Can you work these out from the model? Positions are in its coordinate system, mm. A direction names the side the tool comes from. Round coordinates to 2 decimals unless told otherwise and drop trailing zeros. Write each loop counter-clockwise with the first axis right and the second up, starting at its lowest first coordinate (ties: lowest second). Pieces come first, ordered by that corner, then holes. Notation, with made-up numbers: M 33,-1.5 L 51,-1.5 A22 cw 51,17.5 Z; hole C 85,86.25 d4. An arc over 180 degrees is marked long. Answer as a JSON object with one key per item and string values. Group by question number.
1) Suppose I cut it at A-A, the plane x = 38.13. Write out the boundary of the cut face in (y, z), and give its area (3 significant figures).
2) Please list where these lines run through material, in increasing order: L1, parallel to Z at x = 41.88, y = 36.4; L2, parallel to X at y = 36, z = 3.75; L3, parallel to Y at x = 35.5, z = 24.25. Write a range as [from, to].
3) Suppose I cut it at B-B, the plane x = 50.5. Write out the boundary of the cut face in (y, z).
4) Suppose I cut it at D-D, the plane y = 28. Write out the boundary of the cut face in (x, z).
5) Suppose I cut it at C-C, the plane z = 14.5. Write out the boundary of the cut face in (x, y).
6) I'm going to push flat-ended pins straight in: pin 1 Ø1 at (y, z) = (9.5, 7) entering from -X; pin 2 Ø1.1 at (x, z) = (22.5, 3.5) entering from +Y; pin 3 Ø5 at (y, z) = (19.5, 18) entering from +X. Where does each tip first touch, or does it pass through?
7) On a 3-axis mill with a long thin cutter (end or side, diameter ignored), from which of +Z, -Z, +X, -X, +Y, -Y can I reach the whole of each face in a straight line? I mean faces 1 (the flat face through (3, 37, 3)), 2 (the flat face through (5, 1, 23)), 3 (the flat face through (17, 36, 6.5)), 4 (the flat face through (65, 1, 26)), 5 (the flat face through (25, 2, 14)). Say none if no direction works.
8) If we mould it in two halves opening along Z, with no side actions, what happens to faces 6 (the flat face through (60, 1, 23)), 7 (the flat face through (0, 1, 2)), 8 (the flat face through (32, 16, 28)), 9 (the cylindrical face through (37.589, 0.507, 22.533))? For each: +Z half, -Z half, draft (parallel to the pull), parting line (faces both ways), or undercut.
from build123d import *

# Parameters (mm, degrees)
SKETCH_1_W           = 65
SKETCH_1_H           = 38
EXTRUDE_1_DEPTH      = 28
SKETCH_2_W           = 30
SKETCH_2_H           = 32
CUT_EXTRUDE_1_DEPTH  = 81.330567034
CUT_EXTRUDE_3_REACH  = 82.331
SKETCH_3_R           = 0.75
SKETCH_4_W           = 15
SKETCH_4_H           = 1.5
CUT_EXTRUDE_4_DEPTH  = 30
SKETCH_5_R           = 11
CUT_EXTRUDE_5_DEPTH  = 81.330567034
CUT_EXTRUDE_6_REACH  = 82.331
SKETCH_6_R           = 0.75
CUT_EXTRUDE_7_REACH  = 82.331
SKETCH_7_W           = 8
SKETCH_7_H           = 24.102688632
SKETCH_8_R           = 1.8
CUT_EXTRUDE_8_DEPTH  = 1
CUT_EXTRUDE_START    = -1
SKETCH_9_R           = 1.8
CUT_EXTRUDE_9_DEPTH  = 1
SKETCH_10_W          = 20
SKETCH_10_H          = 1.7
CUT_EXTRUDE_10_DEPTH = 12


with BuildPart() as part:
    # Sketch 1 → Extrude 1 (new body)
    with BuildSketch(Plane.XY):
        with Locations((32.5, 19)):
            Rectangle(SKETCH_1_W, SKETCH_1_H)
    extrude(amount=EXTRUDE_1_DEPTH)

    # Sketch 2 → Cut-Extrude 1 (cut, through all)
    with BuildSketch(Plane.XY.offset(28)):
        with Locations((15, 19)):
            Rectangle(SKETCH_2_W, SKETCH_2_H)
    cut_extrude_1 = extrude(amount=-CUT_EXTRUDE_1_DEPTH, mode=Mode.SUBTRACT)

    # Sketch 3 → Cut-Extrude 3 (cut, up to next)
    with BuildSketch(Plane(origin=(0, 38, 0), x_dir=(1, 0, 0), z_dir=(0, 1, 0)), mode=Mode.PRIVATE) as cut_extrude_3_sk1:
        with Locations(Location((2.42, -3.75, 0), (0, 0, 270))):
            Circle(SKETCH_3_R)
    cut_extrude_3_tool1 = extrude(cut_extrude_3_sk1.sketch, amount=-CUT_EXTRUDE_3_REACH, mode=Mode.PRIVATE) & part.part
    # Sketch 3 → Cut-Extrude 3 (cut, up to next)
    with BuildSketch(Plane(origin=(0, 38, 0), x_dir=(1, 0, 0), z_dir=(0, 1, 0)), mode=Mode.PRIVATE) as cut_extrude_3_sk2:
        with Locations(Location((23.12, -3.75, 0), (0, 0, 270))):
            Circle(SKETCH_3_R)
    cut_extrude_3_tool2 = extrude(cut_extrude_3_sk2.sketch, amount=-CUT_EXTRUDE_3_REACH, mode=Mode.PRIVATE) & part.part
    # Sketch 3 → Cut-Extrude 3 (cut, up to next)
    with BuildSketch(Plane(origin=(0, 38, 0), x_dir=(1, 0, 0), z_dir=(0, 1, 0)), mode=Mode.PRIVATE) as cut_extrude_3_sk3:
        with Locations(Location((23.12, -24.25, 0), (0, 0, 270))):
            Circle(SKETCH_3_R)
    cut_extrude_3_tool3 = extrude(cut_extrude_3_sk3.sketch, amount=-CUT_EXTRUDE_3_REACH, mode=Mode.PRIVATE) & part.part
    # Sketch 3 → Cut-Extrude 3 (cut, up to next)
    with BuildSketch(Plane(origin=(0, 38, 0), x_dir=(1, 0, 0), z_dir=(0, 1, 0)), mode=Mode.PRIVATE) as cut_extrude_3_sk4:
        with Locations(Location((2.42, -24.25, 0), (0, 0, 270))):
            Circle(SKETCH_3_R)
    cut_extrude_3_tool4 = extrude(cut_extrude_3_sk4.sketch, amount=-CUT_EXTRUDE_3_REACH, mode=Mode.PRIVATE) & part.part
    cut_extrude_3_1 = cut_extrude_3_tool1.solids().sort_by_distance((2.42, 38, 3.75))[0]
    add(cut_extrude_3_1, mode=Mode.SUBTRACT)
    cut_extrude_3_2 = cut_extrude_3_tool2.solids().sort_by_distance((23.12, 38, 3.75))[0]
    add(cut_extrude_3_2, mode=Mode.SUBTRACT)
    cut_extrude_3_3 = cut_extrude_3_tool3.solids().sort_by_distance((23.12, 38, 24.25))[0]
    add(cut_extrude_3_3, mode=Mode.SUBTRACT)
    cut_extrude_3_4 = cut_extrude_3_tool4.solids().sort_by_distance((2.42, 38, 24.25))[0]
    add(cut_extrude_3_4, mode=Mode.SUBTRACT)
    cut_extrude_3 = cut_extrude_3_1 + cut_extrude_3_2 + cut_extrude_3_3 + cut_extrude_3_4  # Cut-Extrude 3 as one shape, for the pattern or mirror that repeats it

    # Sketch 4 → Cut-Extrude 4 (cut)
    with BuildSketch(Plane.ZY):
        with Locations((14, 35.75)):
            Rectangle(SKETCH_4_W, SKETCH_4_H)
    cut_extrude_4 = extrude(amount=-CUT_EXTRUDE_4_DEPTH, mode=Mode.SUBTRACT)

    # Sketch 5 → Cut-Extrude 5 (cut, through all)
    with BuildSketch(Plane(origin=(0, 38, 0), x_dir=(1, 0, 0), z_dir=(0, 1, 0))):
        with Locations((-4.5, -14)):
            Circle(SKETCH_5_R)
    cut_extrude_5 = extrude(amount=-CUT_EXTRUDE_5_DEPTH, mode=Mode.SUBTRACT)

    # Sketch 6 → Cut-Extrude 6 (cut, up to next)
    with BuildSketch(Plane.XZ, mode=Mode.PRIVATE) as cut_extrude_6_sk1:
        with Locations(Location((2.42, 3.75, 0), (0, 0, 90))):
            Circle(SKETCH_6_R)
    cut_extrude_6_tool1 = extrude(cut_extrude_6_sk1.sketch, amount=-CUT_EXTRUDE_6_REACH, mode=Mode.PRIVATE) & part.part
    # Sketch 6 → Cut-Extrude 6 (cut, up to next)
    with BuildSketch(Plane.XZ, mode=Mode.PRIVATE) as cut_extrude_6_sk2:
        with Locations(Location((2.42, 24.25, 0), (0, 0, 90))):
            Circle(SKETCH_6_R)
    cut_extrude_6_tool2 = extrude(cut_extrude_6_sk2.sketch, amount=-CUT_EXTRUDE_6_REACH, mode=Mode.PRIVATE) & part.part
    # Sketch 6 → Cut-Extrude 6 (cut, up to next)
    with BuildSketch(Plane.XZ, mode=Mode.PRIVATE) as cut_extrude_6_sk3:
        with Locations(Location((26.87, 24.25, 0), (0, 0, 270))):
            Circle(SKETCH_6_R)
    cut_extrude_6_tool3 = extrude(cut_extrude_6_sk3.sketch, amount=-CUT_EXTRUDE_6_REACH, mode=Mode.PRIVATE) & part.part
    # Sketch 6 → Cut-Extrude 6 (cut, up to next)
    with BuildSketch(Plane.XZ, mode=Mode.PRIVATE) as cut_extrude_6_sk4:
        with Locations(Location((26.87, 3.75, 0), (0, 0, 270))):
            Circle(SKETCH_6_R)
    cut_extrude_6_tool4 = extrude(cut_extrude_6_sk4.sketch, amount=-CUT_EXTRUDE_6_REACH, mode=Mode.PRIVATE) & part.part
    cut_extrude_6_1 = cut_extrude_6_tool1.solids().sort_by_distance((2.42, 0, 3.75))[0]
    add(cut_extrude_6_1, mode=Mode.SUBTRACT)
    cut_extrude_6_2 = cut_extrude_6_tool2.solids().sort_by_distance((2.42, 0, 24.25))[0]
    add(cut_extrude_6_2, mode=Mode.SUBTRACT)
    cut_extrude_6_3 = cut_extrude_6_tool3.solids().sort_by_distance((26.87, 0, 24.25))[0]
    add(cut_extrude_6_3, mode=Mode.SUBTRACT)
    cut_extrude_6_4 = cut_extrude_6_tool4.solids().sort_by_distance((26.87, 0, 3.75))[0]
    add(cut_extrude_6_4, mode=Mode.SUBTRACT)
    cut_extrude_6 = cut_extrude_6_1 + cut_extrude_6_2 + cut_extrude_6_3 + cut_extrude_6_4  # Cut-Extrude 6 as one shape, for the pattern or mirror that repeats it

    # Sketch 7 → Cut-Extrude 7 (cut, up to next)
    with BuildSketch(Plane.XZ, mode=Mode.PRIVATE) as cut_extrude_7_sk1:
        with Locations((9, 14)):
            Rectangle(SKETCH_7_W, SKETCH_7_H)
    cut_extrude_7_tool1 = extrude(cut_extrude_7_sk1.sketch, amount=-CUT_EXTRUDE_7_REACH, mode=Mode.PRIVATE) & part.part
    cut_extrude_7 = cut_extrude_7_tool1.solids().sort_by_distance((9, 0, 14))[0]
    add(cut_extrude_7, mode=Mode.SUBTRACT)

    # Sketch 8 → Cut-Extrude 8 (cut)
    with BuildSketch(Plane(origin=(0, 38, 0), x_dir=(1, 0, 0), z_dir=(0, 1, 0))):
        with Locations(Location((23.12, -3.75, 0), (0, 0, 270))):
            Circle(SKETCH_8_R)
        with Locations((2.42, -3.75)):
            Circle(SKETCH_8_R)
        with Locations((2.42, -24.25)):
            Circle(SKETCH_8_R)
        with Locations(Location((23.12, -24.25, 0), (0, 0, 270))):
            Circle(SKETCH_8_R)
    cut_extrude_8 = extrude(amount=-CUT_EXTRUDE_8_DEPTH, mode=Mode.SUBTRACT)

    # Sketch 9 → Cut-Extrude 9 (cut)
    with BuildSketch(Plane.XZ.offset(CUT_EXTRUDE_START)):
        with Locations((2.42, 24.25)):
            Circle(SKETCH_9_R)
        with Locations(Location((26.87, 24.25, 0), (0, 0, 270))):
            Circle(SKETCH_9_R)
        with Locations(Location((26.87, 3.75, 0), (0, 0, 270))):
            Circle(SKETCH_9_R)
        with Locations((2.42, 3.75)):
            Circle(SKETCH_9_R)
    cut_extrude_9 = extrude(amount=CUT_EXTRUDE_9_DEPTH, mode=Mode.SUBTRACT)

    # Sketch 10 → Cut-Extrude 10 (cut)
    with BuildSketch(Plane.ZY.offset(-13)):
        with Locations((14, 2.15)):
            Rectangle(SKETCH_10_W, SKETCH_10_H)
    cut_extrude_10 = extrude(amount=-CUT_EXTRUDE_10_DEPTH, mode=Mode.SUBTRACT)

    # Mirror 1: Cut-Extrude 1, Cut-Extrude 3, Cut-Extrude 4, Cut-Extrude 5, Cut-Extrude 6, Cut-Extrude 7, Cut-Extrude 8, Cut-Extrude 9, Cut-Extrude 10 across plane
    add(cut_extrude_1.mirror(Plane.ZY.offset(-32.5)), mode=Mode.SUBTRACT)
    add(cut_extrude_3.mirror(Plane.ZY.offset(-32.5)), mode=Mode.SUBTRACT)
    add(cut_extrude_4.mirror(Plane.ZY.offset(-32.5)), mode=Mode.SUBTRACT)
    add(cut_extrude_5.mirror(Plane.ZY.offset(-32.5)), mode=Mode.SUBTRACT)
    add(cut_extrude_6.mirror(Plane.ZY.offset(-32.5)), mode=Mode.SUBTRACT)
    add(cut_extrude_7.mirror(Plane.ZY.offset(-32.5)), mode=Mode.SUBTRACT)
    add(cut_extrude_8.mirror(Plane.ZY.offset(-32.5)), mode=Mode.SUBTRACT)
    add(cut_extrude_9.mirror(Plane.ZY.offset(-32.5)), mode=Mode.SUBTRACT)
    add(cut_extrude_10.mirror(Plane.ZY.offset(-32.5)), mode=Mode.SUBTRACT)


solid = part.part
Results:
{
 "1": {"outline": "M 0,0 L 3,0 L 3,3 L 1,3 L 1,1.95 L 0,1.95 Z; M 0,5.55 L 1,5.55 L 1,4.5 L 3,4.5 L 3,23.5 L 1,23.5 L 1,22.45 L 0,22.45 Z; M 0,26.05 L 1,26.05 L 1,25 L 3,25 L 3,28 L 0,28 Z; M 35,0 L 38,0 L 38,28 L 35,28 L 35,21.5 L 36.5,21.5 L 36.5,6.5 L 35,6.5 Z", "area": "132 mm^2"},
 "2": {"L1": "[0, 3], [4.5, 6.5], [21.5, 23.5], [25, 28]", "L2": "[0, 1.67], [3.17, 22.37], [23.87, 41.13], [42.63, 61.83], [63.33, 65]", "L3": "[0, 3], [35, 38]"},
 "3": {"outline": "M 0,0 L 3,0 L 3,4 L 1.3,4 L 1.3,24 L 3,24 L 3,28 L 0,28 Z; M 35,0 L 38,0 L 38,28 L 35,28 L 35,21.5 L 36.5,21.5 L 36.5,6.5 L 35,6.5 Z"},
 "4": {"outline": "M 30,0 L 35,0 L 35,28 L 30,28 Z"},
 "5": {"outline": "M 6.49,36.5 L 30,36.5 L 30,3 L 25,3 L 25,1.3 L 13,1.3 L 13,0 L 52,0 L 52,1.3 L 40,1.3 L 40,3 L 35,3 L 35,36.5 L 58.51,36.5 L 58.51,38 L 6.49,38 Z"},
 "6": {"pin 1": "x = 30", "pin 2": "y = 37", "pin 3": "x = 35"},
 "7": {"face 1": "+Y", "face 2": "-Y", "face 3": "-X", "face 4": "+Z, -Z, +X, +Y, -Y", "face 5": "none"},
 "8": {"face 6": "undercut", "face 7": "draft", "face 8": "+Z half", "face 9": "undercut"}
}
